from build123d import *

# Parameters (mm, degrees)
SKETCH1_W           = 76.354636869
SKETCH1_H           = 38
SKETCH1_R           = 4.55
BOSS_EXTRUDE1_DEPTH = 3
SKETCH2_W           = 76.354636869
SKETCH2_H           = 38
BOSS_EXTRUDE2_DEPTH = 0.6
SKETCH3_R           = 3.5
CUT_EXTRUDE1_DEPTH  = 0.4
SKETCH4_R           = 2.5
BOSS_EXTRUDE3_DEPTH = 3.6


with BuildPart() as part:
    # Sketch1 → Boss-Extrude1 (new body)
    with BuildSketch(Plane.XY):
        with Locations((22.177318435, 0)):
            Rectangle(SKETCH1_W, SKETCH1_H)
        Circle(SKETCH1_R, mode=Mode.SUBTRACT)
    extrude(amount=BOSS_EXTRUDE1_DEPTH)

    # Sketch2 → Boss-Extrude2 (add)
    with BuildSketch(Plane(origin=(0, 0, 3), x_dir=(-1, 0, 0), z_dir=(0, 0, -1))):
        with Locations((-22.177318435, 0)):
            Rectangle(SKETCH2_W, SKETCH2_H)
    extrude(amount=-BOSS_EXTRUDE2_DEPTH)

    # Sketch3 → Cut-Extrude1 (cut)
    with BuildSketch(Plane(origin=(0, 0, 3), x_dir=(-1, 0, 0), z_dir=(0, 0, -1))):
        Circle(SKETCH3_R)
    extrude(amount=-CUT_EXTRUDE1_DEPTH, mode=Mode.SUBTRACT)

    # Sketch4 → Boss-Extrude3 (add)
    with BuildSketch(Plane(origin=(0, 0, 0), x_dir=(-1, 0, 0), z_dir=(0, 0, -1))):
        Polygon((-15.354636869, -19), (-46.354636869, -60), (-60.354636869, -19), align=None)
        with Locations((-35.354636869, -24)):
            Circle(SKETCH4_R, mode=Mode.SUBTRACT)
    extrude(amount=-BOSS_EXTRUDE3_DEPTH)


solid = part.part
CAD build for the part. Positions are in the model's coordinates, mm. A direction names the side the tool comes from. Coordinates: 2 decimals unless noted, no trailing zeros. Write each loop counter-clockwise with the first axis right and the second up, starting at its lowest first coordinate (ties: lowest second). Pieces come first, ordered by that corner, then holes. Notation, with made-up numbers: M 54.5,45.5 L 90.5,45.5 A25 cw 90.5,64.5 Z; hole C 25,-13 d7. An arc over 180 degrees is marked long. Answer as a JSON object with one key per item and string values. Group by question number.
1) Tool access for faces 1 (the face through (30, -11, 0)), 2 (the face through (0, 0, 3.4)), 3 (the face through (0, -19, 2)): list every direction of +Z, -Z, +X, -X, +Y, -Y with a clear straight run to the whole face (end or side of a thin tool).
2) Saw through at D-D (x = -8). Write the cut outline in (y, z).
3) Pin check, flat tips, straight feed: pin 1 Ø1.5 at (x, z) = (13.5, 1) entering from -Y; pin 2 Ø5.5 at (x, y) = (0, 1) entering from -Z; pin 3 Ø4.5 at (x, y) = (35.35, -24) entering from -Z. Stop position of each tip, or through.
4) Saw through at A-A (y = 0). Write the cut outline in (x, z).
5) Saw through at C-C (x = 1.5). Write the cut outline in (y, z).
6) Mould opens along Y. For faces 4 (the face through (-16, 0, 2)), 5 (the face through (30.638, -39.213, 1.775)), 6 (the face through (-0.99, -4.44, 1.48)) say: +Y half, -Y half, draft (parallel to the pull), parting line (faces both ways), or undercut.
7) Wall check: line 1 (Y direction, x = 0, z = 3.15); line 2 (Y direction, x = -4, z = 3.2); line 3 (Y direction, x = 0, z = 1.25). Give the ranges that are in metal, low to high. Write a range as from..to.
8) Saw through at B-B (y = -24). Write the cut outline in (x, z), plus the area to 3 significant figures.
Values follow:
{
 "1": {"face 1": "-Z, +X, -X, +Y, -Y", "face 2": "-Z", "face 3": "+Z, -Z, -X, -Y"},
 "2": {"outline": "M -19,0 L 19,0 L 19,3.6 L -19,3.6 Z"},
 "3": {"pin 1": "stops at y = -19", "pin 2": "stops at z = 3", "pin 3": "passes through"},
 "4": {"outline": "M -16,0 L -4.55,0 L -4.55,3 L -3.5,3 L -3.5,3.4 L 3.5,3.4 L 3.5,3 L 4.55,3 L 4.55,0 L 60.35,0 L 60.35,3.6 L -16,3.6 Z"},
 "5": {"outline": "M -19,0 L -4.3,0 L -4.3,3 L -3.16,3 L -3.16,3.4 L 3.16,3.4 L 3.16,3 L 4.3,3 L 4.3,0 L 19,0 L 19,3.6 L -19,3.6 Z"},
 "6": {"face 4": "draft", "face 5": "-Y half", "face 6": "undercut"},
 "7": {"line 1": "y = -19..-3.5, 3.5..19", "line 2": "y = -19..19", "line 3": "y = -19..-4.55, 4.55..19"},
 "8": {"outline": "M 19.14,0 L 32.85,0 L 32.85,3.6 L 19.14,3.6 Z; M 37.85,0 L 58.65,0 L 58.65,3.6 L 37.85,3.6 Z", "area": "124 mm2"}
}
